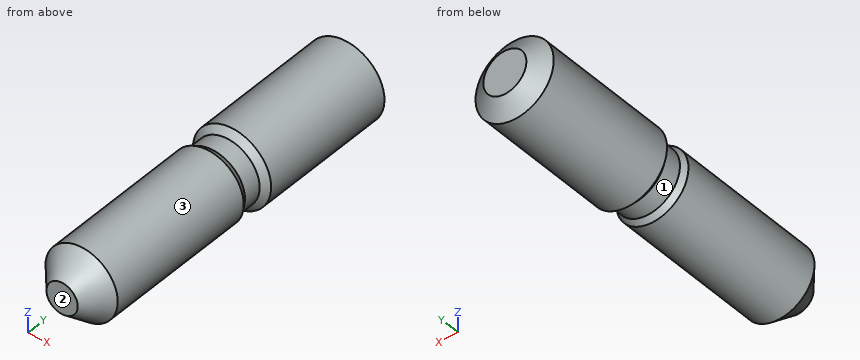
```python
from build123d import *


with BuildPart() as part:
    # Sketch1 → Motor_reductora_husillo (revolve)
    with BuildSketch(Plane.XY, mode=Mode.PRIVATE) as motor_reductora_husillo_sk:
        Polygon((0, 0), (3.575, 0), (6.5, -2), (6.5, -25.2), (5.4, -26.2), (5.4, -29.2), (6, -30.2), (6, -56), (2.6, -60), (0, -60), align=None)
    revolve(motor_reductora_husillo_sk.sketch.rotate(Axis((0, -64, 0), (0, 1, 0)), 90), axis=Axis((0, -64, 0), (0, 1, 0)))


solid = part.part
```
For this review, take the finished solid that the model builds, in its own axes (mm). Face numbers are marked on the shaded views. Round coordinates to 2 decimals unless told otherwise and drop trailing zeros. Write each loop counter-clockwise with the first axis right and the second up, starting at its lowest first coordinate (ties: lowest second). Pieces come first, ordered by that corner, then holes. Notation, with made-up numbers: M 33.5,-35 L 84.5,-35 A31 cw 84.5,4 Z; hole C -3.75,82 d10. An arc over 180 degrees is marked long. One line per item, written item: value. Start each with the question number.
(1) Insertion check: pin 1 (6 mm diameter, centred on y = -24, z = -4, fed in from +X); pin 2 (6 mm diameter, centred on y = -27, z = 4, fed in from +X); pin 3 (1.5 mm diameter, centred on y = -9.5, z = 3, fed in from +X). Each pin has a flat end and moves straight along its axis. Give the tip position at first contact, or say it passes through.
(2) We need section B-B (x = 0). Give the boundary of the cut face in (y, z) (3 decimals).
(3) We need section A-A (z = 0). Give the boundary of the cut face in (x, y) (3 decimals), and give its area (3 significant figures).
(4) The part is to be moulded in two halves that separate along Y. For the marked faces 1, 2 and 3, say which applies: released by +Y, released by -Y, zero draft, split by the parting line, or undercut.
(5) We need section C-C (y = -7). Give the boundary of the cut face in (x, z), and give its area (3 significant figures).
(6) We need section D-D (y = -51). Give the boundary of the cut face in (x, z).
(7) Wall thickness on line 1 (X direction, y = -2.5, z = 2.5); line 2 (Y direction, x = -4.25, z = -3.75); line 3 (Y direction, x = 5.5, z = -2): over which ranges is each line inside the solid? List them lowest first.
Result:
1. pin 1: x = 6.42
1. pin 2: x = 6.3
1. pin 3: x = 6.1
2. outline: M -60,-2.6 L -56,-6 L -30.2,-6 L -29.2,-5.4 L -26.2,-5.4 L -25.2,-6.5 L -2,-6.5 L 0,-3.575 L 0,3.575 L -2,6.5 L -25.2,6.5 L -26.2,5.4 L -29.2,5.4 L -30.2,6 L -56,6 L -60,2.6 Z
3. outline: M -6.5,-25.2 L -5.4,-26.2 L -5.4,-29.2 L -6,-30.2 L -6,-56 L -2.6,-60 L 2.6,-60 L 6,-56 L 6,-30.2 L 5.4,-29.2 L 5.4,-26.2 L 6.5,-25.2 L 6.5,-2 L 3.575,0 L -3.575,0 L -6.5,-2 Z
3. area: 721 mm²
4. face 1: undercut
4. face 2: released by -Y
4. face 3: zero draft
5. outline: C 0,0 d13
5. area: 133 mm²
6. outline: C 0,0 d12
7. line 1: -6 to 6
7. line 2: -56.39 to -29.65, -25.96 to -1.43
7. line 3: -56.17 to -29.95, -25.79 to -1.56
